from build123d import *

# Parameters (mm, degrees)
F1_DEPTH = 4
F2_R     = 1
F3_DEPTH = 1
F4_R     = 0.5
F5_DEPTH = 25


with BuildPart() as f1:
    # F0 (on Top) → F1 (new body)
    with BuildSketch(Plane.XY):
        with BuildLine():
            Line((0, 4), (0, 0))
            Line((0, 0), (4, 0))
            ThreePointArc((4, 0), (4.292893, 0.707107), (5, 1))
            Line((5, 1), (5, 4))
            Line((5, 4), (0, 4))
        make_face()
    extrude(amount=-F1_DEPTH)

    # F2 (on Front) → F3 (join)
    with BuildSketch(Plane.XZ):
        with Locations((2, -2)):
            Circle(F2_R)
    extrude(amount=F3_DEPTH)

    # F4 (on face) → F5 (cut)
    with BuildSketch(Plane.YZ.offset(5)):
        with Locations((2.5, -1.5)):
            Circle(F4_R)
    extrude(amount=-F5_DEPTH, mode=Mode.SUBTRACT)


solid = f1.part
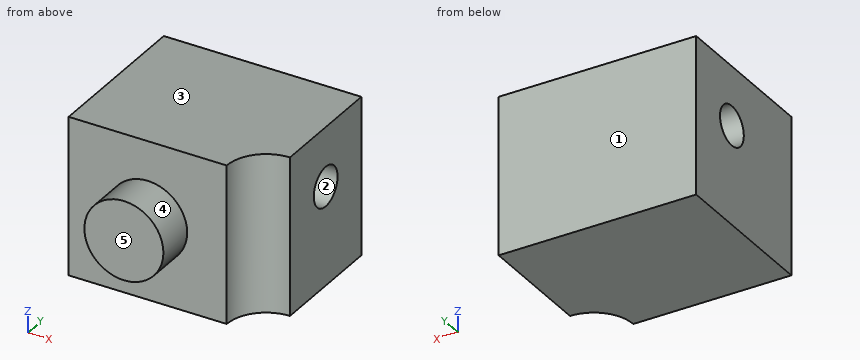
Model file for the job. Use its own axes, mm. Face numbers are marked on the shaded views. A direction names the side the tool comes from. Give positions to 0.01 mm unless a question says otherwise; leave off trailing zeros. Write each loop counter-clockwise with the first axis right and the second up, starting at its lowest first coordinate (ties: lowest second). Pieces come first, ordered by that corner, then holes. Notation, with made-up numbers: (3.25, 49) - (37.25, 49) arc R18 ccw to (37.25, 66) - close; hole circle Ø1 at (46.25, 85). An arc over 180 degrees is marked (long way). Answer as CSV lines item,"result".
1. Band-saw the part on C-C (z = -1.5). Write the cut outline in (x, y), and give its area (3 significant figures).
Responses:
outline,"(0, 0) - (1.13, 0) - (1.13, -1) - (2.87, -1) - (2.87, 0) - (4, 0) arc R1 cw to (5, 1) - (5, 2) - (0, 2) - close; (0, 3) - (5, 3) - (5, 4) - (0, 4) - close"
area,"15.9 mm2"
2. Pin check, flat tip, straight feed: pin 1 (1 mm diameter, centred on y = 0, z = -1, fed in from +X). Stop position of the tip, or through.
Responses:
pin 1,"stops at x = 4.13"
3. Band-saw the part on D-D (x = 1.4). Write the cut outline in (y, z).
Responses:
outline,"(-1, -2.8) - (0, -2.8) - (0, -4) - (4, -4) - (4, 0) - (0, 0) - (0, -1.2) - (-1, -1.2) - close; hole circle Ø1 at (2.5, -1.5)"
4. 3-axis set-ups, long thin cutter, end or side, ignore diameter. For the marked faces 4 and 5: which of +Z, -Z, +X, -X, +Y, -Y reach the whole face in a straight line?
Responses:
face 4,"-Y"
face 5,"+Z, -Z, +X, -X, -Y"
5. Band-saw the part on A-A (x = 2). Write the cut outline in (y, z), and give its area (3 significant figures).
Responses:
outline,"(-1, -3) - (0, -3) - (0, -4) - (4, -4) - (4, 0) - (0, 0) - (0, -1) - (-1, -1) - close; hole circle Ø1 at (2.5, -1.5)"
area,"17.2 mm2"
6. Drill centre lines: L1, parallel to Z at x = 2.65, y = 2.5; L2, parallel to Y at x = 0.5, z = -2.45; L3, parallel to Y at x = 3.15, z = -1.65. Where is each one in solid material? Low to high. Write a range as [from, to].
Responses:
L1,"z = [-4, -2], [-1, 0]"
L2,"y = [0, 4]"
L3,"y = [0, 2.02], [2.98, 4]"
7. Band-saw the part on B-B (y = 2.5). Write the cut outline in (x, z), and give its area (3 significant figures).
Responses:
outline,"(0, -4) - (5, -4) - (5, -2) - (0, -2) - close; (0, -1) - (5, -1) - (5, 0) - (0, 0) - close"
area,"15.0 mm2"
8. Two-plate mould, pull along Z, no slides. Class the marked faces 1, 2 and 3: +Z half, -Z half, draft (parallel to the pull), parting line (faces both ways), or undercut.
Responses:
face 1,"draft"
face 2,"undercut"
face 3,"+Z half"
